from build123d import *

# Parameters (mm, degrees)
CROQUIS1_R                 = 4
CROQUIS1_R_2               = 2.6
SALIENTE_EXTRUIR2_DEPTH    = 10.2
CORTAR_EXTRUIR3_DEPTH      = 11.2
CROQUIS4_R                 = 2
CORTAR_EXTRUIR4_DEPTH      = 12.5
CORTAR_EXTRUIR4_DEPTH_BACK = 32.5


with BuildPart() as part:
    # Croquis1 → Saliente-Extruir2 (new body)
    with BuildSketch(Plane.XY):
        with BuildLine():
            Line((-10, 0), (10, 0))
            Line((10, 0), (10, 5))
            Line((10, 5), (19.881270341, 11.098702893))
            ThreePointArc((19.881270341, 11.098702893), (21.48800967, 14.28568517), (19.37161624, 17.15959299))
            Line((19.37161624, 17.15959299), (2.5, 24))
            Line((2.5, 24), (-2.5, 24))
            Line((-2.5, 24), (-19.37161624, 17.15959299))
            ThreePointArc((-19.37161624, 17.15959299), (-21.48800967, 14.28568517), (-19.881270341, 11.098702893))
            Line((-19.881270341, 11.098702893), (-10, 5))
            Line((-10, 5), (-10, 0))
        make_face()
        with Locations((0, 14)):
            Circle(CROQUIS1_R, mode=Mode.SUBTRACT)
        with Locations((16.05, 14)):
            Circle(CROQUIS1_R_2, mode=Mode.SUBTRACT)
        with Locations((-16.05, 14)):
            Circle(CROQUIS1_R_2, mode=Mode.SUBTRACT)
    extrude(amount=SALIENTE_EXTRUIR2_DEPTH)

    # Croquis3 → Cortar-Extruir3 (cut, through all)
    with BuildSketch(Plane.XY.offset(10.2)):
        with BuildLine():
            Line((-1, 0), (-1, 10.127016654))
            ThreePointArc((-1, 10.127016654), (0, 10), (1, 10.127016654))
            Line((1, 10.127016654), (1, 0))
            Line((1, 0), (-1, 0))
        make_face()
    extrude(amount=-CORTAR_EXTRUIR3_DEPTH, mode=Mode.SUBTRACT)

    # Croquis4 → Cortar-Extruir4 (cut, two sides)
    with BuildSketch(Plane(origin=(10, 0, 0), x_dir=(0, 0, -1), z_dir=(1, 0, 0))) as cortar_extruir4_sk:
        with Locations((-5.1, 2.5)):
            Circle(CROQUIS4_R)
    extrude(amount=CORTAR_EXTRUIR4_DEPTH, mode=Mode.SUBTRACT)
    extrude(cortar_extruir4_sk.sketch, amount=-CORTAR_EXTRUIR4_DEPTH_BACK, mode=Mode.SUBTRACT)


solid = part.part
Read the model definition and answer for the solid it produces. Units are mm, in the model's axes. A direction names the side the tool comes from. Round coordinates to 2 decimals unless told otherwise and drop trailing zeros. Write each loop counter-clockwise with the first axis right and the second up, starting at its lowest first coordinate (ties: lowest second). Pieces come first, ordered by that corner, then holes. Notation, with made-up numbers: M -39,88.25 L -15,88.25 A16 cw -15,95.25 Z; hole C 60,89 d11. An arc over 180 degrees is marked long. Use a Markdown table: item, result.
1) The part is cut by section D-D (x = 18). Write down the section's boundary in (y, z).
Answers follow:
| item | result |
|---|---|
| outline | M 9.94,0 L 12.28,0 L 12.28,10.2 L 9.94,10.2 Z; M 15.72,0 L 17.72,0 L 17.72,10.2 L 15.72,10.2 Z |
2) Straight lines are drawn through the part: line 1 along X through (y, z) = (14.75, 9.5); line 2 along Y through (x, z) = (3.5, 5.1); line 3 along X through (y, z) = (17, 8). For each, find the intervals that lie inside material, in ascending order. Write a range as [from, to].
Answers follow:
| item | result |
|---|---|
| line 1 | x = [-21.42, -18.54], [-13.56, -3.93], [3.93, 13.56], [18.54, 21.42] |
| line 2 | y = [0, 0.5], [4.5, 12.06], [15.94, 23.59] |
| line 3 | x = [-19.71, -2.65], [2.65, 19.71] |
3) Flat-ended cylindrical pins translate along their axes: pin 1 (3 mm diameter, centred on y = 5.5, z = 7, fed in from -X); pin 2 (5 mm diameter, centred on y = 17, z = 3, fed in from -X); pin 3 (3 mm diameter, centred on y = 2.5, z = 6, fed in from +X). Find the tip coordinate at first contact, or state that the pin passes through.
Answers follow:
| item | result |
|---|---|
| pin 1 | stops at x = -13.24 |
| pin 2 | stops at x = -21.46 |
| pin 3 | stops at x = 10 |
4) A tool of negligible diameter and unlimited length cuts with its end or side. For faces 4 (the flat face through (1, 5, 5)), 5 (the flat face through (-6, 0, 5)), 6 (the flat face through (-10, 4.8, 5)), from which of +Z, -Z, +X, -X, +Y, -Y can it reach the whole face along a straight path? Write none if from no direction.
Answers follow:
| item | result |
|---|---|
| face 4 | +Z, -Z, -Y |
| face 5 | +Z, -Z, +X, -X, -Y |
| face 6 | +Z, -Z, -X, -Y |
5) The part is cut by section C-C (z = 2.25). Write down the section's boundary in (x, y).
Answers follow:
| item | result |
|---|---|
| outline | M -19.88,11.1 L -10,5 L -10,0 L -1,0 L -1,10.13 A4 cw long 1,10.13 L 1,0 L 10,0 L 10,5 L 19.88,11.1 A3.41 ccw 19.37,17.16 L 2.5,24 L -2.5,24 L -19.37,17.16 A3.41 ccw Z; hole C -16.05,14 d5.2; hole C 16.05,14 d5.2 |
6) For a pull along Y with two mould halves and no side action, classify faces 1 (the cylindrical face through (-16.61, 11.46, 5.03)), 2 (the flat face through (10, 0.2, 5)), 3 (the flat face through (0, 24, 5)) as pulls with the +Y half, pulls with the -Y half, needs draft (parallel to the pull), parting line crosses it, or undercut.
Answers follow:
| item | result |
|---|---|
| face 1 | undercut |
| face 2 | needs draft |
| face 3 | pulls with the +Y half |
7) The part is cut by section B-B (y = 14). Write down the section's boundary in (x, z).
Answers follow:
| item | result |
|---|---|
| outline | M -21.5,0 L -18.65,0 L -18.65,10.2 L -21.5,10.2 Z; M -13.45,0 L -4,0 L -4,10.2 L -13.45,10.2 Z; M 4,0 L 13.45,0 L 13.45,10.2 L 4,10.2 Z; M 18.65,0 L 21.5,0 L 21.5,10.2 L 18.65,10.2 Z |
8) The part is cut by section A-A (z = 5.1). Write down the section's boundary in (x, y).
Answers follow:
| item | result |
|---|---|
| outline | M -19.88,11.1 L -10,5 L -10,4.5 L -1,4.5 L -1,10.13 A4 cw long 1,10.13 L 1,4.5 L 10,4.5 L 10,5 L 19.88,11.1 A3.41 ccw 19.37,17.16 L 2.5,24 L -2.5,24 L -19.37,17.16 A3.41 ccw Z; M -10,0 L -1,0 L -1,0.5 L -10,0.5 Z; M 1,0 L 10,0 L 10,0.5 L 1,0.5 Z; hole C -16.05,14 d5.2; hole C 16.05,14 d5.2 |
